Input: part model. Units: mm. Frame: model coordinates. A direction names the side the tool comes from. Round coordinates to 2 decimals unless told otherwise and drop trailing zeros. Loops run counter-clockwise (first coordinate to the right, second up) from the corner with the lowest first, then second, coordinate; pieces in that order, holes last. Notation, with made-up numbers: M 45,21.25 L 85,21.25 A23 ccw 85,53.25 Z; hole C 5,10.25 d4. An arc over 180 degrees is marked long. Return JSON: item names as keys, results as strings. Group by question number.
1) Contact query for flat-ended pins moving along their axis: P1, Ø16, axis at y = 27.5, z = 3.5, coming from the +X side; P2, Ø10, axis at y = 38, z = -6.5, coming from the +X side; P3, Ø1, axis at y = 6.5, z = 11.5, coming from the -X side. Output: stop coordinate, or through.
2) Section A-A (x = 22). Output: boundary loops of the cut face in (y, z), plus the area to 3 significant figures.
3) Access query for faces 4 (the face through (30, 45, 0)), 5 (the face through (41, 10, 0)), 6 (the face through (42, 0, 0)). Directions: +Z, -Z, +X, -X, +Y, -Y. A direction counts if a zero-diameter tool reaches every point of the face in a straight line with its end or side. Return the directions, or none.
4) Mould query, pull axis X, two halves, no side actions, for faces 1 (the face through (11, 50, 0)), 2 (the face through (40, 5, 0)), 3 (the face through (10, 30, 0)). Classes: +X half, -X half, draft (parallel to the pull), parting line (faces both ways), or undercut.
5) Section B-B (z = -1). Output: boundary loops of the cut face in (x, y), plus the area to 3 significant figures.
6) Material intervals for line 1 (Z direction, x = 30, y = 7.25); line 2 (Y direction, x = 22.5, z = 7.5); line 3 (Y direction, x = 14.5, z = -6), sorted ascending. Write a range as from..to.
7) Section C-C (y = 29.5). Output: boundary loops of the cut face in (x, z), plus the area to 3 significant figures.
8) Section D-D (z = 16). Output: boundary loops of the cut face in (x, y).
from build123d import *

# Parameters (mm, degrees)
EXTRUDE_THIN1_DEPTH = 20
FILLET1_R           = 20
FILLET2_R           = 10
FILLET3_RADIUS      = 20
FILLET3_LENGTH      = 10
FILLET4_RADIUS      = 20
FILLET4_LENGTH      = 10
SKETCH2_R           = 10
CUT_EXTRUDE1_DEPTH  = 68.082039325


with BuildPart() as part:
    # Sketch1 → Extrude-Thin1 (new, symmetric)
    with BuildSketch(Plane.XY):
        Polygon((50, 0), (0, 0), (0, 50), (30, 50), (30, 40), (10, 40), (10, 10), (50, 10), align=None)
    extrude(amount=EXTRUDE_THIN1_DEPTH, both=True)

    # Fillet1
    fillet1_edges = [part.edges().sort_by_distance(p)[0] for p in [
        (0, 0, 0),
    ]]
    fillet(fillet1_edges, radius=FILLET1_R)

    # Fillet2
    fillet2_edges = [part.edges().sort_by_distance(p)[0] for p in [
        (10, 10, 0),
    ]]
    fillet(fillet2_edges, radius=FILLET2_R)

    # Fillet3: full round fillet: the end face becomes a half cylinder, R = half its width
    fillet3_face = Plane((30, 45, 0), x_dir=(0, -1, 0), z_dir=(1, 0, 0))  # on the end face: x along it, z out of the body
    fillet3_slab = fillet3_face.offset(-FILLET3_RADIUS / 2) * Box(FILLET3_LENGTH, 2 * FILLET3_RADIUS, FILLET3_RADIUS, mode=Mode.PRIVATE)  # the body's end, R deep
    fillet3_round = Plane((10, 45, 0), x_dir=(1, 0, 0), z_dir=(0, -1, 0)) * Cylinder(FILLET3_RADIUS, FILLET3_LENGTH, mode=Mode.PRIVATE)  # its axis R under the face
    add(fillet3_slab - fillet3_round, mode=Mode.SUBTRACT)

    # Fillet4: full round fillet: the end face becomes a half cylinder, R = half its width
    fillet4_face = Plane((50, 5, 0), x_dir=(0, -1, 0), z_dir=(1, 0, 0))  # on the end face: x along it, z out of the body
    fillet4_slab = fillet4_face.offset(-FILLET4_RADIUS / 2) * Box(FILLET4_LENGTH, 2 * FILLET4_RADIUS, FILLET4_RADIUS, mode=Mode.PRIVATE)  # the body's end, R deep
    fillet4_round = Plane((30, 5, 0), x_dir=(1, 0, 0), z_dir=(0, -1, 0)) * Cylinder(FILLET4_RADIUS, FILLET4_LENGTH, mode=Mode.PRIVATE)  # its axis R under the face
    add(fillet4_slab - fillet4_round, mode=Mode.SUBTRACT)

    # Sketch2 → Cut-Extrude1 (cut, through all)
    with BuildSketch(Plane(origin=(0, 10, 0), x_dir=(1, 0, 0), z_dir=(0, 1, 0))):
        with Locations(Location((30, 0, 0), (0, 0, 180))):
            Circle(SKETCH2_R)
    extrude(amount=-CUT_EXTRUDE1_DEPTH, mode=Mode.SUBTRACT)


solid = part.part
Returned:
{
 "1": {"P1": "stops at x = 10.01", "P2": "stops at x = 29.91", "P3": "stops at x = 4.8"},
 "2": {"outline": "M 0,-20 L 10,-20 L 10,-6 L 0,-6 Z; M 0,6 L 10,6 L 10,20 L 0,20 Z; M 40,-16 L 50,-16 L 50,16 L 40,16 Z", "area": "600 mm^2"},
 "3": {"face 4": "+X, +Y", "face 5": "+Z, -Z, +X", "face 6": "+Z, -Z, +X, -X, -Y"},
 "4": {"face 1": "draft", "face 2": "undercut", "face 3": "+X half"},
 "5": {"outline": "M 0,20 A20 ccw 20,0 L 20.05,0 L 20.05,10 L 20,10 A10 cw 10,20 L 10,40 L 29.97,40 L 29.97,50 L 0,50 Z; M 39.95,0 L 49.97,0 L 49.97,10 L 39.95,10 Z", "area": "836 mm^2"},
 "6": {"line 1": "z = -20..-10, 10..20", "line 2": "y = 0..10, 40..50", "line 3": "y = 0.77..11.65, 40..50"},
 "7": {"outline": "M 0,-20 L 10,-20 L 10,20 L 0,20 Z", "area": "400 mm^2"},
 "8": {"outline": "M 0,20 A20 ccw 20,0 L 42,0 L 42,10 L 20,10 A10 cw 10,20 L 10,40 L 22,40 L 22,50 L 0,50 Z"}
}
